Answer from the drawing. Dimensions are ordinates in mm from the lowest x, y and z of the part. Give positions to 0.01 mm unless a question says otherwise; leave off trailing zeros. Loops run counter-clockwise (first coordinate to the right, second up) from the corner with the lowest first, then second, coordinate; pieces in that order, holes last.
(1) Straight lines are drawn through the part: probe 1 along Z at (x, y) = (45, 2.85) (1 decimal); probe 2 along Z at (x, y) = (15, 1.45) (1 decimal). For each, find the intervals that lie inside material, in ascending order.
(2) This flat-tipped pin is pushed along its axis until it touches: P1, Ø5, axis at x = 43.12, z = 75.26, coming from the -Y side. Where does it stop, or does it pass through?
(3) Find section C-C, the plane y = 2.1. Write down the section's boundary in (x, z).
(4) Find section B-B, the plane x = 13. Write down the section's boundary in (y, z) (1 decimal).
(5) Find section A-A, the plane z = 76.5. Write down the section's boundary in (x, y) (1 decimal).
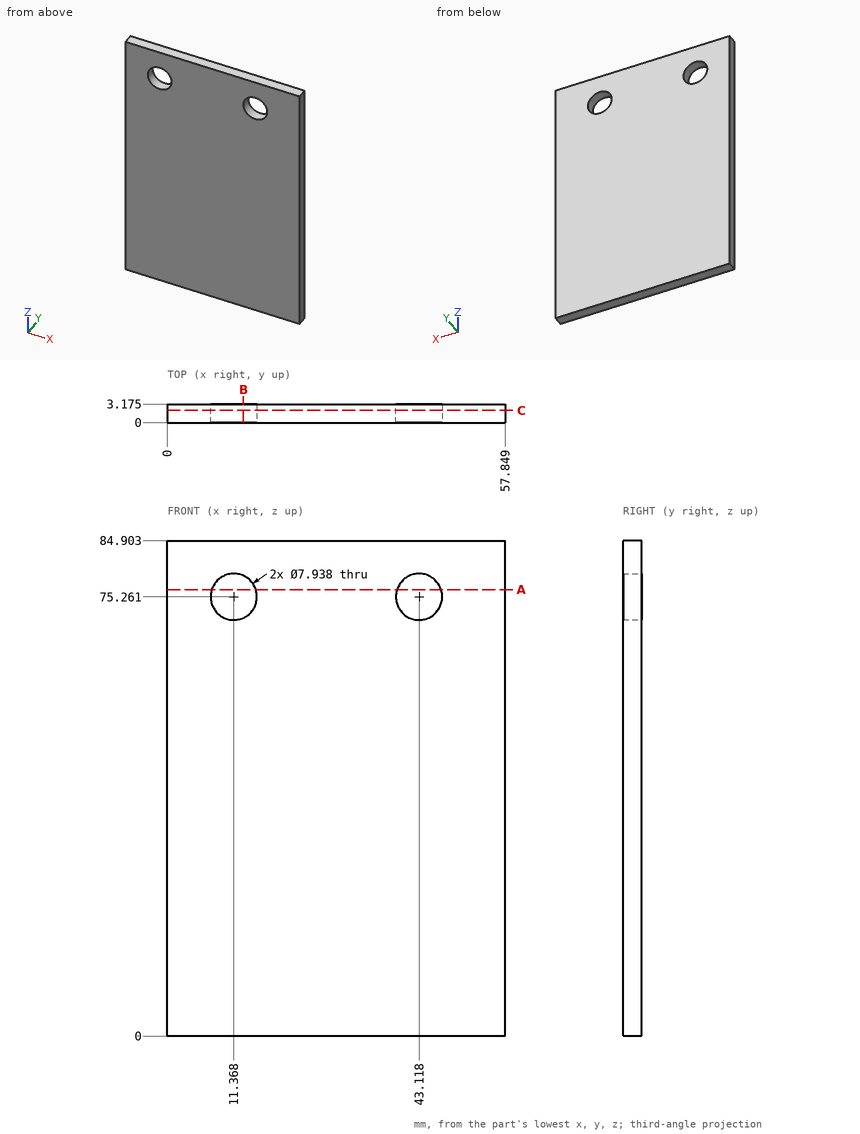
Entries:
1. probe 1: z = 0 to 71.8, 78.8 to 84.9
1. probe 2: z = 0 to 73.7, 76.9 to 84.9
2. P1: passes through
3. outline: (0, 0) - (57.85, 0) - (57.85, 84.9) - (0, 84.9) - close; hole circle Ø7.94 at (11.37, 75.26); hole circle Ø7.94 at (43.12, 75.26)
4. outline: (0, 0) - (3.2, 0) - (3.2, 71.6) - (0, 71.6) - close; (0, 78.9) - (3.2, 78.9) - (3.2, 84.9) - (0, 84.9) - close
5. outline: (0, 0) - (7.6, 0) - (7.6, 3.2) - (0, 3.2) - close; (15.1, 0) - (39.3, 0) - (39.3, 3.2) - (15.1, 3.2) - close; (46.9, 0) - (57.8, 0) - (57.8, 3.2) - (46.9, 3.2) - close
